Autodesk Inventor part; units mm, degrees
ref_plane "YZ Plane" through (0, 0, 0) normal (1, 0, 0) x (0, 1, 0)
ref_plane "XZ Plane" through (0, 0, 0) normal (0, 1, 0) x (-1, 0, 0)
ref_plane "XY Plane" through (0, 0, 0) normal (0, 0, 1) x (1, 0, 0)
sketch "Sketch1" plane through (0, 0, 0) normal (1, 0, 0) x (0, 1, 0)
  circle A0 centre (0, 0) radius 9
  circle A1 centre (0, 0) radius 5
  dimension "d0" = 18
  dimension "d1" = 10
extrude "Extrusion1" add sketch "Sketch1" along normal blind 13.9
sketch "Sketch2" plane through (0, 0, 0) normal (-1, 0, 0) x (0, 0, 1)
  circle A0 centre (0, 0) radius 7
  point P0 (0, 7)
  dimension "d4" = 14
hole "Hole1" at (0, 7, 0) direction (1, 0, 0) diameter 1.6 depth 5
pattern_circular "Circular Pattern1" count 4 over 360 about axis through (0, 0, 0) along (1, 0, 0) of "Hole1"
thread "Thread1"
thread "Thread2"
thread "Thread3"
thread "Thread4"
properties part number "sample-transfer_rod" material "ABS Plastic orange"
Verification items for the finished model (mm, model axes). A direction names the side the tool comes from. Give positions to 0.01 mm unless a question says otherwise; leave off trailing zeros. Write each loop counter-clockwise with the first axis right and the second up, starting at its lowest first coordinate (ties: lowest second). Pieces come first, ordered by that corner, then holes. Notation, with made-up numbers: (56.5, -20.5) - (83.5, -20.5) arc R21 cw to (83.5, -13.5) - close; hole circle Ø10 at (22.5, -12.75). An arc over 180 degrees is marked (long way). Answer as CSV lines item,"result". Start each with the question number.
1. Sectioned sample at A-A (y = 0). Record the boundary of the cut face in (x, z).
2. Sectioned sample at D-D (z = -6.5). Record the boundary of the cut face in (x, y), then the cut area to 3 significant figures.
3. Draft check along Y on faces 1 (the face through (6.853, -1.172, -8.923)), 2 (the face through (2.535, -6.207, 0.104)), 3 (the face through (0, 4, -4)). Enter one of: pulls with the +Y half, pulls with the -Y half, needs draft (parallel to the pull), parting line crosses it, or undercut.
4. Depth check by flat-ended pin: pin 1 (6 mm diameter, centred on x = 1.5, y = -5.5, fed in from -Z); pin 2 (2 mm diameter, centred on x = 8, z = 5.5, fed in from +Y); pin 3 (1.3 mm diameter, centred on y = -7, z = 0, fed in from -X). Enter the tip coordinate at first touch or a pass-through.
5. Thickness scan on line 1 (Z direction, x = 1.05, y = 0); line 2 (Z direction, x = 2.75, y = 3); line 3 (Y direction, x = 2.8, z = 7). Record the ranges inside material, lowest first.
6. Sectioned sample at B-B (x = 4.25). Record the boundary of the cut face in (y, z), then the cut area to 3 significant figures.
7. Set-up check for faces 4 (the face through (5, 7, 0)), 5 (the face through (6.85, -1.08, 4.88)): record each of +Z, -Z, +X, -X, +Y, -Y from which the full face is reachable in a straight line by a thin tool's end or side.
Derived:
1,outline,"(0, -9) - (13.9, -9) - (13.9, -5) - (0, -5) - (0, -6.2) - (5, -6.2) - (5, -7.8) - (0, -7.8) - close; (0, 5) - (13.9, 5) - (13.9, 9) - (0, 9) - (0, 7.8) - (5, 7.8) - (5, 6.2) - (0, 6.2) - close"
2,outline,"(0, -6.22) - (13.9, -6.22) - (13.9, 6.22) - (0, 6.22) - (0, 0.62) - (5, 0.62) - (5, -0.62) - (0, -0.62) - close"
2,area,"167 mm²"
3,face 1,"parting line crosses it"
3,face 2,"undercut"
3,face 3,"needs draft"
4,pin 1,"z = -8.65"
4,pin 2,"y = 7.79"
4,pin 3,"x = 5"
5,line 1,"-9 to -7.8, -6.2 to -5, 5 to 6.2, 7.8 to 9"
5,line 2,"-8.49 to -4, 4 to 8.49"
5,line 3,"-5.66 to -0.8, 0.8 to 5.66"
6,outline,"circle Ø18 at (0, 0); hole circle Ø1.6 at (-7, 0); hole circle Ø10 at (0, 0); hole circle Ø1.6 at (0, -7); hole circle Ø1.6 at (0, 7); hole circle Ø1.6 at (7, 0)"
6,area,"168 mm²"
7,face 4,"-X"
7,face 5,"+X, -X"
